Verification items for the finished model (mm, model axes). A direction names the side the tool comes from. Give positions to 0.01 mm unless a question says otherwise; leave off trailing zeros. Loops run counter-clockwise (first coordinate to the right, second up) from the corner with the lowest first, then second, coordinate; pieces in that order, holes last. Notation, with made-up numbers: M -22,16 L 21,16 A31 cw 21,53 Z; hole C -8.5,57.5 d1. An arc over 180 degrees is marked long. Use a Markdown table: item, result.
Autodesk Inventor part; units mm, degrees
ref_plane "YZ Plane" through (0, 0, 0) normal (1, 0, 0) x (0, 1, 0)
ref_plane "XZ Plane" through (0, 0, 0) normal (0, 1, 0) x (-1, 0, 0)
ref_plane "XY Plane" through (0, 0, 0) normal (0, 0, 1) x (1, 0, 0)
sketch "スケッチ1" plane through (0, 0, 0) normal (0, 0, 1) x (1, 0, 0)
  line L0 (-100, -100) -> (100, -100)
  line L1 (100, -100) -> (100, 100)
  line L2 (100, 100) -> (-100, 100)
  line L3 (-100, 100) -> (-100, -100)
  line L4 (-100, -100) -> (100, 100) construction
  line L5 (100, -100) -> (-100, 100) construction
  point P0 (0, 0)
  dimension "d0" = 200
extrude "押し出し1" add sketch "スケッチ1" along normal blind 300
sketch "スケッチ2" plane through (0, 0, 0) normal (1, 0, 0) x (0, 1, 0)
  line L0 (0, 300) -> (14, 300)
  line L1 (14, 300) -> (14, 340)
  line L2 (9, 345) -> (0, 345)
  line L3 (0, 345) -> (0, 300)
  line L4 (100, 300) -> (-100, 300)
  line L5 (0, 330) -> (60, 330)
  line L6 (60, 330) -> (60, 325)
  line L7 (60, 325) -> (0, 325)
  line L8 (0, 325) -> (0, 330)
  arc A0 (14, 340) -> (9, 345) centre (9, 340) ccw
  point P0 (0, 0)
  dimension "d3" = 14
  dimension "d4" = 45
  dimension "d5" = 5
  dimension "d6" = 60
  dimension "d7" = 15
  dimension "d8" = 5
  dimension "d10" = 25
revolve "回転1" add sketch "スケッチ2" angle 360 about axis through (0, 0, 345) along (0, 0, -1)
properties part number "Wind Trubin Engine"
(1) Cross-section at B-B on y = 34.5. Record the cut outline in (x, z), then the cut area to 3 significant figures.
Results below:
| item | result |
|---|---|
| outline | M -100,0 L 100,0 L 100,300 L -100,300 Z; M -49.09,325 L 49.09,325 L 49.09,330 L -49.09,330 Z |
| area | 60,500 mm^2 |
(2) Material ranges on line 1 (Z direction, x = 36, y = -30); line 2 (Z direction, x = -85.5, y = 56), recorded low to high.
Results below:
| item | result |
|---|---|
| line 1 | 0 to 300, 325 to 330 |
| line 2 | 0 to 300 |
(3) Cross-section at A-A on x = -36. Record the cut outline in (y, z), then the cut area to 3 significant figures.
Results below:
| item | result |
|---|---|
| outline | M -100,0 L 100,0 L 100,300 L -100,300 Z; M -48,325 L 48,325 L 48,330 L -48,330 Z |
| area | 60,500 mm^2 |
(4) Set-up check for faces 1 (the cylindrical face through (2.64, -59.94, 327.46)), 2 (the cylindrical face through (5.362, 12.932, 312.675)), 3 (the flat face through (0, 0, 345)): record each of +Z, -Z, +X, -X, +Y, -Y from which the full face is reachable in a straight line by a thin tool's end or side.
Results below:
| item | result |
|---|---|
| face 1 | +Z |
| face 2 | none |
| face 3 | +Z, +X, -X, +Y, -Y |
(5) Cross-section at C-C on x = 0. Record the cut outline in (y, z).
Results below:
| item | result |
|---|---|
| outline | M -100,0 L 100,0 L 100,300 L 14,300 L 14,325 L 60,325 L 60,330 L 14,330 L 14,340 A5 ccw 9,345 L -9,345 A5 ccw -14,340 L -14,330 L -60,330 L -60,325 L -14,325 L -14,300 L -100,300 Z |
(6) Draft check along Z on faces 4 (the flat face through (1, 100, 148)), 5 (the flat face through (-1, 24, 300)), 6 (the flat face through (-1, 1, 0)), 7 (the flat face through (14.2, -0.8, 325)). Enter one of: +Z half, -Z half, draft (parallel to the pull), parting line (faces both ways), or undercut.
Results below:
| item | result |
|---|---|
| face 4 | draft |
| face 5 | undercut |
| face 6 | -Z half |
| face 7 | undercut |
(7) Gauge pin test, flat end, axial feed: P1, Ø1, axis at x = -63.5, y = -39, coming from the +Z side. Record the tip position at first contact, or that the pin passes through.
Results below:
| item | result |
|---|---|
| P1 | z = 300 |
